from build123d import *
from OCP.BRepFilletAPI import BRepFilletAPI_MakeChamfer

# Parameters (mm, degrees)
SCHIZZO1_W               = 37
SCHIZZO1_H               = 21.5
ESTRUSIONE1_DEPTH        = 85
SCHIZZO6_W               = 73
SCHIZZO6_H               = 23.639461627
TAGLIO_ESTRUSIONE4_DEPTH = 84
SCHIZZO7_R               = 5.5
ESTRUSIONE4_DEPTH        = 73
SMUSSO1_SIZE             = 3
SMUSSO1_SIZE2            = 0.803847577
RACCORDO1_R              = 4
SCHIZZO8_R               = 45
TAGLIO_ESTRUSIONE5_DEPTH = 96.395230489
SCHIZZO9_R               = 3
TAGLIO_ESTRUSIONE6_DEPTH = 8.5


with BuildPart() as part:
    # Schizzo1 → Estrusione1 (new body)
    with BuildSketch(Plane.XY):
        with Locations((18.5, 10.75)):
            Rectangle(SCHIZZO1_W, SCHIZZO1_H)
    extrude(amount=ESTRUSIONE1_DEPTH)

    # Schizzo6 → Taglio-Estrusione4 (cut)
    with BuildSketch(Plane(origin=(37, 0, 0), x_dir=(0, 0, -1), z_dir=(1, 0, 0))):
        with Locations((-42.5, 20.319730814)):
            Rectangle(SCHIZZO6_W, SCHIZZO6_H)
    extrude(amount=-TAGLIO_ESTRUSIONE4_DEPTH, mode=Mode.SUBTRACT)

    # Schizzo7 → Estrusione4 (add)
    with BuildSketch(Plane.XY.offset(6)):
        with Locations(Location((5, 17, 0), (0, 0, 155.380022671))):
            Circle(SCHIZZO7_R)
        with Locations(Location((17.5, 17, 0), (0, 0, 125.096801228))):
            Circle(SCHIZZO7_R)
        with Locations(Location((30, 17, 0), (0, 0, 125.096801228))):
            Circle(SCHIZZO7_R)
    extrude(amount=ESTRUSIONE4_DEPTH)

    # Smusso1: one chamfer whose edges measure the first distance from different faces: ONE call of the kernel's chamfer builder (chamfer() names one face for all edges)
    smusso1_edges_1 = [part.edges().sort_by_distance(p)[0] for p in [
        (37, 21.5, 3),
    ]]
    smusso1_side_1 = [part.faces().sort_by_distance(p)[0] for p in [
        (18.5, 21.5, 3),
    ]]
    smusso1_edges_2 = [part.edges().sort_by_distance(p)[0] for p in [
        (37, 21.5, 82),
    ]]
    smusso1_side_2 = [part.faces().sort_by_distance(p)[0] for p in [
        (18.5, 21.5, 82),
    ]]
    smusso1 = BRepFilletAPI_MakeChamfer(part.part.solid().wrapped)
    for e in smusso1_edges_1:
        smusso1.Add(SMUSSO1_SIZE, SMUSSO1_SIZE2, e.wrapped, smusso1_side_1[0].wrapped)  # the first distance lies on this face
    for e in smusso1_edges_2:
        smusso1.Add(SMUSSO1_SIZE, SMUSSO1_SIZE2, e.wrapped, smusso1_side_2[0].wrapped)  # the first distance lies on this face
    add(Compound.cast(smusso1.Shape()), mode=Mode.REPLACE)

    # Raccordo1
    # the kernel refuses this fillet: 4 mm, written as the material it takes off along each edge
    with BuildSketch(Plane(origin=(0, 21.5, -10), x_dir=(1, 0, 0), z_dir=(0, 0, 1))) as raccordo1_piece_1:
        with BuildLine():
            CenterArc((RACCORDO1_R, -RACCORDO1_R), RACCORDO1_R, 90, 90)
            Line((0, -RACCORDO1_R), (0, 0))
            Line((0, 0), (RACCORDO1_R, 0))
        make_face()
    extrude(amount=16, mode=Mode.SUBTRACT)
    with BuildSketch(Plane(origin=(0, 21.5, 79), x_dir=(0, -1, 0), z_dir=(0, 0, 1))) as raccordo1_piece_2:
        with BuildLine():
            CenterArc((RACCORDO1_R, RACCORDO1_R), RACCORDO1_R, 180, 90)
            Line((0, RACCORDO1_R), (0, 0))
            Line((0, 0), (RACCORDO1_R, 0))
        make_face()
    extrude(amount=16, mode=Mode.SUBTRACT)

    # Schizzo8 → Taglio-Estrusione5 (cut, through all)
    with BuildSketch(Plane.XY.offset(85)):
        with Locations((-24.5, -24.5)):
            Circle(SCHIZZO8_R)
    extrude(amount=-TAGLIO_ESTRUSIONE5_DEPTH, mode=Mode.SUBTRACT)

    # Schizzo9 → Taglio-Estrusione6 (cut)
    with BuildSketch(Plane.XZ):
        with Locations(Location((23, 75.5, 0), (0, 0, 270))):
            Circle(SCHIZZO9_R)
        with Locations(Location((23, 9.5, 0), (0, 0, 270))):
            Circle(SCHIZZO9_R)
    extrude(amount=-TAGLIO_ESTRUSIONE6_DEPTH, mode=Mode.SUBTRACT)


solid = part.part
Check sheet for the modelled part. Datum: model origin and axes. Units: mm. A direction names the side the tool comes from. Coordinates: 2 decimals unless noted, no trailing zeros. Write each loop counter-clockwise with the first axis right and the second up, starting at its lowest first coordinate (ties: lowest second). Pieces come first, ordered by that corner, then holes.
Item 1: Access from +Z, -Z, +X, -X, +Y, -Y to the whole of each face (thin tool, end or side, straight path). Record for faces 1 (the face through (2.7, 21.5, 6)), 2 (the face through (23, 13, 79)), 3 (the face through (0, 15, 82)), 4 (the face through (21.2, 4.2, 77.9)).
Numbers:
face 1: -Z, -X, +Y
face 2: none
face 3: +Z, -X, +Y, -Y
face 4: -Y
Item 2: Cross-section at B-B on y = 7.5. Record the boundary of the cut face in (x, z).
Numbers:
outline: (7.14, 0) - (37, 0) - (37, 85) - (7.14, 85) - close; hole circle Ø6 at (23, 9.5); hole circle Ø6 at (23, 75.5)
Item 3: Cross-section at A-A on x = 17.5. Record the boundary of the cut face in (y, z).
Numbers:
outline: (0, 0) - (21.5, 0) - (21.5, 6) - (22.5, 6) - (22.5, 79) - (21.5, 79) - (21.5, 85) - (0, 85) - close; hole (8.5, 6) - (11.5, 6) - (11.5, 79) - (8.5, 79) - close
Item 4: Depth check by flat-ended pin: pin 1 Ø1.8 at (x, z) = (19.5, 82.5) entering from +Y; pin 2 Ø0.5 at (x, y) = (30.5, 22) entering from +Z; pin 3 Ø8 at (x, z) = (27, 10) entering from +Y; pin 4 Ø8 at (y, z) = (9, 65) entering from -X. Enter the tip coordinate at first touch or a pass-through.
Numbers:
pin 1: stops at y = 21.5
pin 2: stops at z = 79
pin 3: stops at y = 22.5
pin 4: stops at x = 1.23
Item 5: Cross-section at C-C on z = 75.5. Record the boundary of the cut face in (x, y), then the cut area to 3 significant figures.
Numbers:
outline: circle Ø11 at (5, 17); (6.09, 8.5) arc R45 cw to (13.25, 0) - (20, 0) - (20, 8.5) - close; circle Ø11 at (17.5, 17); circle Ø11 at (30, 17); (26, 0) - (37, 0) - (37, 8.5) - (26, 8.5) - close
area: 464 mm2
Item 6: Mould release check, pull along Z, two halves, no side actions. Record for faces 5 (the face through (1.203, 20.359, 81.958)), 6 (the face through (22, 8.5, 43)), 7 (the face through (2.7, 21.5, 79)): released by +Z, released by -Z, zero draft, split by the parting line, or undercut.
Numbers:
face 5: zero draft
face 6: undercut
face 7: released by +Z
Item 7: Scan lines: probe 1 along X at (y, z) = (18.5, 77.5); probe 2 along Z at (x, y) = (3.5, 11.5); probe 3 along Y at (x, z) = (23.5, 43.5). Record each from-to range of solid material in increasing order.
Numbers:
probe 1: x = -0.29 to 10.29, 12.21 to 22.79, 24.71 to 35.29
probe 2: z = 0 to 6, 79 to 85
probe 3: y = 0 to 8.5
Item 8: Cross-section at D-D on x = 2. Record the boundary of the cut face in (y, z).
Numbers:
outline: (11.87, 0) - (20.96, 0) - (20.96, 6) - (21.61, 6) - (21.61, 79) - (20.96, 79) - (20.96, 85) - (11.87, 85) - (11.87, 79) - (12.39, 79) - (12.39, 6) - (11.87, 6) - close
